Autodesk Fusion 360 part; units mm, degrees
sketch "Sketch1" plane through (0, 0, 0) normal (0, 0, 1) x (1, 0, 0)
  line L0 (-50, 22.5) -> (50, 22.5)
  line L1 (50, 22.5) -> (50, -22.5)
  line L2 (50, -22.5) -> (-50, -22.5)
  line L3 (-50, -22.5) -> (-50, 22.5)
  line L4 (-50, 22.5) -> (50, -22.5) construction
  dimension "d1" = 100
  dimension "d2" = 45
extrude "Extrude1" add sketch "Sketch1" along normal blind 5
sphere "SpherePrimitive1" add diameter 25 placed x (1, 0, 0) y (0, 1, 0) z (0, 0, 1) at (0, 0, 5)
box "BoxPrimitive1" cut length 45 width 100 height 15 placed x (0, 1, 0) y (1, 0, 0) z (0, 0, -1) at (-50, -22.5, 0)
sketch "Sketch5" plane through (0, 0, 5) normal (0, 0, 1) x (1, 0, 0)
  circle A0 centre (0, 0) radius 12.5
  line L0 (-50, -22.5) -> (50, -22.5)
  line L1 (50, -22.5) -> (50, 22.5)
  line L2 (50, 22.5) -> (-50, 22.5)
  line L3 (-50, 22.5) -> (-50, -22.5)
  line L4 (39, -8.6603) -> (46.5, -4.3301)
  line L5 (46.5, -4.3301) -> (46.5, 4.3301)
  line L6 (46.5, 4.3301) -> (39, 8.6603)
  line L7 (39, 8.6603) -> (31.5, 4.3301)
  line L8 (31.5, 4.3301) -> (31.5, -4.3301)
  line L9 (31.5, -4.3301) -> (39, -8.6603)
  line L10 (12.5, 0) -> (31.5, 0) construction
  line L11 (0, 0) -> (50, 0) construction
  line L12 (-12.5, 0) -> (-31.5, 0) construction
  circle A1 centre (-39, 0) radius 7.5
  point P0 (39, 0)
  dimension "d16" = 19
  dimension "d17" = 15
  dimension "d18" = 19
  dimension "d19" = 15
extrude "Extrude3" add sketch "Sketch5" along normal blind 15 draft -15 contours L4 L5 L6 L7 L8 L9 | A1
sketch "Sketch9" plane through (0, 0, 20) normal (0, 0, 1) x (1, 0, 0)
  circle A0 centre (-39, 0) radius 3.4808
  line L0 (-39, 3.4808) -> (-39, -3.4808)
  point P0 (-39, 0)
revolve "Revolve1" add sketch "Sketch9" angle 180 about axis through (-39, 3.4808, 20) along (0, -1, 0) contours A0 L0 picked at (-38.2402, 0.8769)
chamfer "Chamfer1" distance 1 angle 45 4 edges at (0, -22.5, 5) (50, 0, 5) (0, 22.5, 5) (-50, 0, 5)
Model file for the job. Use its own axes, mm. A direction names the side the tool comes from. Coordinates: 2 decimals unless noted, no trailing zeros. Order: outer loops, then holes, each group sorted by start corner. A loop starts at its lowest first (then second) coordinate and runs counter-clockwise, first axis right, second up. Notation, with made-up numbers: (-4.75, 4.5) -> (20.25, 4.5) arc R18 cw to (20.25, 33.5) -> close; hole circle Ø2 at (37.25, 17.5). An arc over 180 degrees is marked (long way). Return JSON: item names as keys, results as strings.
Item 1: Slice it at D-D (z = 18.75). Write the cut outline in (x, y).
Model answer:
{"outline": "circle Ø7.63 at (-39, 0); (35.18, -2.2) -> (39, -4.41) -> (42.82, -2.2) -> (42.82, 2.2) -> (39, 4.41) -> (35.18, 2.2) -> close"}
Item 2: Wall check: line 1 along X through (y, z) = (-4, 9.5); line 2 along Z through (x, y) = (-41, 13); line 3 along X through (y, z) = (-6.5, 10.25). Give the ranges that are in metal, low to high. Write a range as from..to.
Model answer:
{"line 1": "x = -43.86..-34.14, -10.95..10.95, 33.34..44.66", "line 2": "z = 0..5", "line 3": "x = -9.3..9.3, 38.07..39.93"}
Item 3: Slice it at A-A (z = 6.25). Write the cut outline in (x, y), then the cut area to 3 significant figures.
Model answer:
{"outline": "circle Ø14.33 at (-39, 0); circle Ø24.87 at (0, 0); (31.83, -4.14) -> (39, -8.27) -> (46.17, -4.14) -> (46.17, 4.14) -> (39, 8.27) -> (31.83, 4.14) -> close", "area": "825 mm²"}
Item 4: Mould opens along X. For faces 1 (the face through (-12, 5, 5)), 2 (the face through (-50, 0, 2)), 3 (the face through (42.035, 5.136, 10.728)), 4 (the face through (33.035, 0.061, 10.728)) say: pulls with the +X half, pulls with the -X half, needs draft (parallel to the pull), parting line crosses it, or undercut.
Model answer:
{"face 1": "undercut", "face 2": "pulls with the -X half", "face 3": "pulls with the +X half", "face 4": "undercut"}
Item 5: 3-axis set-ups, long thin cutter, end or side, ignore diameter. For faces 5 (the face through (39, 0, 20)), 6 (the face through (36.07, 5.196, 10.728)), 7 (the face through (35.965, -5.136, 10.728)): which of +Z, -Z, +X, -X, +Y, -Y reach the whole face in a straight line?
Model answer:
{"face 5": "+Z, +X, +Y, -Y", "face 6": "+Z, +Y", "face 7": "+Z, -Y"}
Item 6: Slice it at B-B (y = -16). Write the cut outline in (x, z).
Model answer:
{"outline": "(-50, 0) -> (50, 0) -> (50, 4) -> (49, 5) -> (-49, 5) -> (-50, 4) -> close"}
Item 7: Pin check, flat tips, straight feed: P1, Ø1.5, axis at x = -22.5, y = 1.5, coming from the +Z side; P2, Ø1, axis at x = -12, z = 12, coming from the -Y side; P3, Ø10, axis at x = 0.5, y = -10, coming from the +Z side; P4, Ø2, axis at x = -36.5, z = 6.5, coming from the -Y side. Stop position of each tip, or through.
Model answer:
{"P1": "stops at z = 5", "P2": "passes through", "P3": "stops at z = 16.45", "P4": "stops at y = -7.06"}
Item 8: Slice it at C-C (x = 28.5). Write the cut outline in (y, z).
Model answer:
{"outline": "(-22.5, 0) -> (22.5, 0) -> (22.5, 4) -> (21.5, 5) -> (-21.5, 5) -> (-22.5, 4) -> close"}
